Geometry: final body of the model. Coordinates: model frame, mm. Face numbers are marked on the shaded views. Give positions to 0.01 mm unless a question says otherwise; leave off trailing zeros. Loops run counter-clockwise (first coordinate to the right, second up) from the corner with the lowest first, then second, coordinate; pieces in that order, holes last.
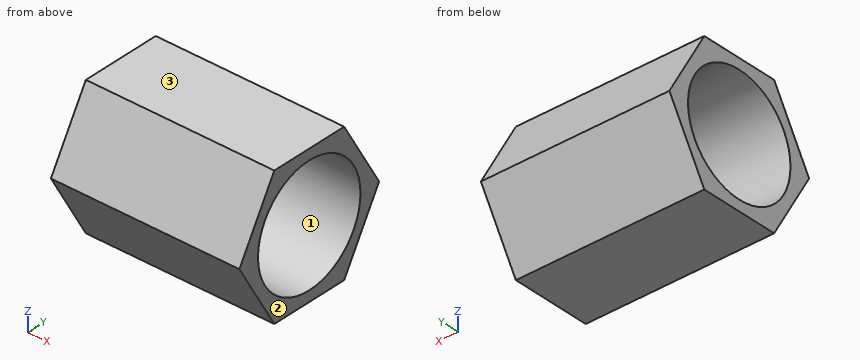
from build123d import *

# Parameters (mm, degrees)
SCHNITT_LINEAR_AUSTRAGEN2_DEPTH = 26.980762114
KREISMUSTER1_COUNT              = 6


with BuildPart() as part:
    # Skizze2 → Rotation1 (revolve)
    with BuildSketch(Plane.XY, mode=Mode.PRIVATE) as rotation1_sk:
        Polygon((-15, 13.5), (-14.598076211, 15), (14.598076211, 15), (15, 13.5), (15, 9.315), (-15, 9.315), align=None)
    revolve(rotation1_sk.sketch.rotate(Axis((-12.825745381, 0, 0), (1, 0, 0)), 90), axis=Axis((-12.825745381, 0, 0), (1, 0, 0)))

    # Skizze3 → Schnitt-Linear austragen2 (cut, symmetric)
    with BuildSketch(Plane(origin=(0, 0, 0), x_dir=(0, 0, -1), z_dir=(1, 0, 0))):
        with BuildLine():
            Line((11, 10.198039027), (11, -10.198039027))
            ThreePointArc((11, -10.198039027), (15, 0), (11, 10.198039027))
        make_face()
    schnitt_linear_austragen2 = extrude(amount=SCHNITT_LINEAR_AUSTRAGEN2_DEPTH, both=True, mode=Mode.SUBTRACT)

    # Kreismuster1: Schnitt-Linear austragen2 ×6 about axis
    kreismuster1_axis = Axis((0, 0, 0), (1, 0, 0))
    for i in range(1, KREISMUSTER1_COUNT):
        add(schnitt_linear_austragen2.rotate(kreismuster1_axis, i * 360 / KREISMUSTER1_COUNT), mode=Mode.SUBTRACT)


solid = part.part
Item 1: Section query B-B on x = 7. Return loops of the section in (y, z) (3 decimals), plus the area to 3 significant figures.
Values follow:
outline: (-12.702, 0) - (-6.351, -11) - (6.351, -11) - (12.702, 0) - (6.351, 11) - (-6.351, 11) - close; hole circle Ø18.63 at (0, 0)
area: 147 mm2
Item 2: Pin query (flat end, axial travel): pin 1 (1.5 mm diameter, centred on x = -8, z = 3.5, fed in from -Y); pin 2 (5 mm diameter, centred on x = -8, z = 5, fed in from +Y); pin 3 (1 mm diameter, centred on x = 0.5, z = 8, fed in from -Y). Return the tip coordinate at first contact, or that it passes through.
Values follow:
pin 1: stops at y = -11.11
pin 2: stops at y = 11.26
pin 3: stops at y = -8.37
Item 3: Section query C-C on z = -3.25. Return loops of the section in (x, y), plus the area to 3 significant figures.
Values follow:
outline: (-15, -10.83) - (15, -10.83) - (15, -8.73) - (-15, -8.73) - close; (-15, 8.73) - (15, 8.73) - (15, 10.83) - (-15, 10.83) - close
area: 126 mm2
Item 4: Draft query along Z for the marked faces 1, 2 and 3. Return one class per face: +Z half, -Z half, draft (parallel to the pull), parting line (faces both ways), or undercut.
Values follow:
face 1: undercut
face 2: draft
face 3: +Z half
Item 5: Section query A-A on y = 0. Return loops of the section in (x, z) (3 decimals).
Values follow:
outline: (-15, -11) - (15, -11) - (15, -9.315) - (-15, -9.315) - close; (-15, 9.315) - (15, 9.315) - (15, 11) - (-15, 11) - close
Item 6: Ray query, probe 1 along Z at (x, y) = (-6, 0.25); probe 2 along Y at (x, z) = (8, -2.75); probe 3 along Z at (x, y) = (5, -3). Return the intervals inside material, ascending.
Values follow:
probe 1: z = -11 to -9.31, 9.31 to 11
probe 2: y = -11.11 to -8.9, 8.9 to 11.11
probe 3: z = -11 to -8.82, 8.82 to 11
Item 7: Section query D-D on y = 11. Return loops of the section in (x, z).
Values follow:
outline: (-15, -2.95) - (15, -2.95) - (15, 2.95) - (-15, 2.95) - close
